Here's how the part is built. I have some questions about the finished solid (model axes, mm). A direction names the side the tool comes from. Coordinates: 2 decimals unless noted, no trailing zeros. Write each loop counter-clockwise with the first axis right and the second up, starting at its lowest first coordinate (ties: lowest second). Pieces come first, ordered by that corner, then holes. Notation, with made-up numbers: M -30,33 L 26,33 A23 ccw 26,48 Z; hole C -16,25 d3. An arc over 180 degrees is marked long. Use a Markdown table: item, result.
```python
from build123d import *

# Parameters (mm, degrees)
F1_DEPTH = 152.4
F2_W     = 12.7
F2_H     = 25.4
F3_DEPTH = 203.2


with BuildPart() as f1:
    # F0 (on Right) → F1 (new body)
    with BuildSketch(Plane.YZ):
        Polygon((-3.175, -76.2), (0, -76.2), (0, 0), (39.37, 0), (39.37, -38.1), (42.545, -38.1), (42.545, 3.175), (-3.175, 3.175), align=None)
    extrude(amount=F1_DEPTH)

    # F2 (on face) → F3 (join)
    with BuildSketch(Plane.XZ.offset(3.175)):
        with Locations((47.625, -36.054839)):
            Rectangle(F2_W, F2_H)
        with Locations((104.775, -36.054839)):
            Rectangle(F2_W, F2_H)
    extrude(amount=F3_DEPTH)


solid = f1.part
```
1. Suppose I cut it at C-C on x = 26. Write out the boundary of the cut face in (y, z) (3 decimals), and give its area (3 significant figures).
Answers follow:
| item | result |
|---|---|
| outline | M -3.175,-76.2 L 0,-76.2 L 0,0 L 39.37,0 L 39.37,-38.1 L 42.545,-38.1 L 42.545,3.175 L -3.175,3.175 Z |
| area | 508 mm2 |
2. Suppose I cut it at B-B on z = -12.5. Write out the boundary of the cut face in (x, y) (3 decimals).
Answers follow:
| item | result |
|---|---|
| outline | M 0,-3.175 L 152.4,-3.175 L 152.4,0 L 0,0 Z; M 0,39.37 L 152.4,39.37 L 152.4,42.545 L 0,42.545 Z |
3. Will these pins go through, and if not, where does the flat tip stop? pin 1 Ø11.5 at (x, z) = (66.5, -12) entering from -Y (3 decimals); pin 2 Ø6.5 at (x, y) = (49, -128) entering from -Z; pin 3 Ø7.5 at (y, z) = (-133, -36.5) entering from -X (3 decimals); pin 4 Ø10 at (y, z) = (-82, -18) entering from +X.
Answers follow:
| item | result |
|---|---|
| pin 1 | stops at y = -3.175 |
| pin 2 | stops at z = -48.75 |
| pin 3 | stops at x = 41.275 |
| pin 4 | passes through |
4. We'd pull the mould along Y, two halves only. Please class faces 4 (the face through (105, -206.375, -36)), 5 (the face through (75, 19, 0)), 6 (the face through (75, 20, 3.175)): +Y half, -Y half, draft (parallel to the pull), parting line (faces both ways), or undercut.
Answers follow:
| item | result |
|---|---|
| face 4 | -Y half |
| face 5 | undercut |
| face 6 | draft |
5. Which directions (+Z, -Z, +X, -X, +Y, -Y) give clear straight access to the entire face, cutting with the end or side of a thin tool? Please do faces 1 (the face through (41.275, -103, -36)), 2 (the face through (53.975, -103, -36)), 3 (the face through (48, -103, -48.755)).
Answers follow:
| item | result |
|---|---|
| face 1 | +Z, -Z, -X, -Y |
| face 2 | +Z, -Z, -Y |
| face 3 | -Z, +X, -X, -Y |
6. I need wall thicknesses on probe 1 along Y at (x, z) = (11, -4) (3 decimals); probe 2 along X at (y, z) = (-138, -31) (3 decimals); probe 3 along Y at (x, z) = (98.5, -28) (3 decimals). Which ranges of each line are inside material? Lowest first, please.
Answers follow:
| item | result |
|---|---|
| probe 1 | y = -3.175 to 0, 39.37 to 42.545 |
| probe 2 | x = 41.275 to 53.975, 98.425 to 111.125 |
| probe 3 | y = -206.375 to 0, 39.37 to 42.545 |
7. Suppose I cut it at A-A on y = -43. Write out the boundary of the cut face in (x, z) (3 decimals).
Answers follow:
| item | result |
|---|---|
| outline | M 41.275,-48.755 L 53.975,-48.755 L 53.975,-23.355 L 41.275,-23.355 Z; M 98.425,-48.755 L 111.125,-48.755 L 111.125,-23.355 L 98.425,-23.355 Z |
8. Suppose I cut it at D-D on z = -43.5. Write out the boundary of the cut face in (x, y) (3 decimals), and give its area (3 significant figures).
Answers follow:
| item | result |
|---|---|
| outline | M 0,-3.175 L 41.275,-3.175 L 41.275,-206.375 L 53.975,-206.375 L 53.975,-3.175 L 98.425,-3.175 L 98.425,-206.375 L 111.125,-206.375 L 111.125,-3.175 L 152.4,-3.175 L 152.4,0 L 0,0 Z |
| area | 5,650 mm2 |
